Job drawing, mm, ordinate dimensions from the low corner. One solid piece. Round coordinates to 2 decimals unless told otherwise and drop trailing zeros. Order: outer loops, then holes, each group sorted by start corner. A loop starts at its lowest first (then second) coordinate and runs counter-clockwise, first axis right, second up. Notation, with made-up numbers: (62, 73.25) -> (96, 73.25) arc R7 cw to (96, 84.25) -> close; hole circle Ø10 at (52.5, 32.5). An arc over 180 degrees is marked (long way). Write item = value, one per line.
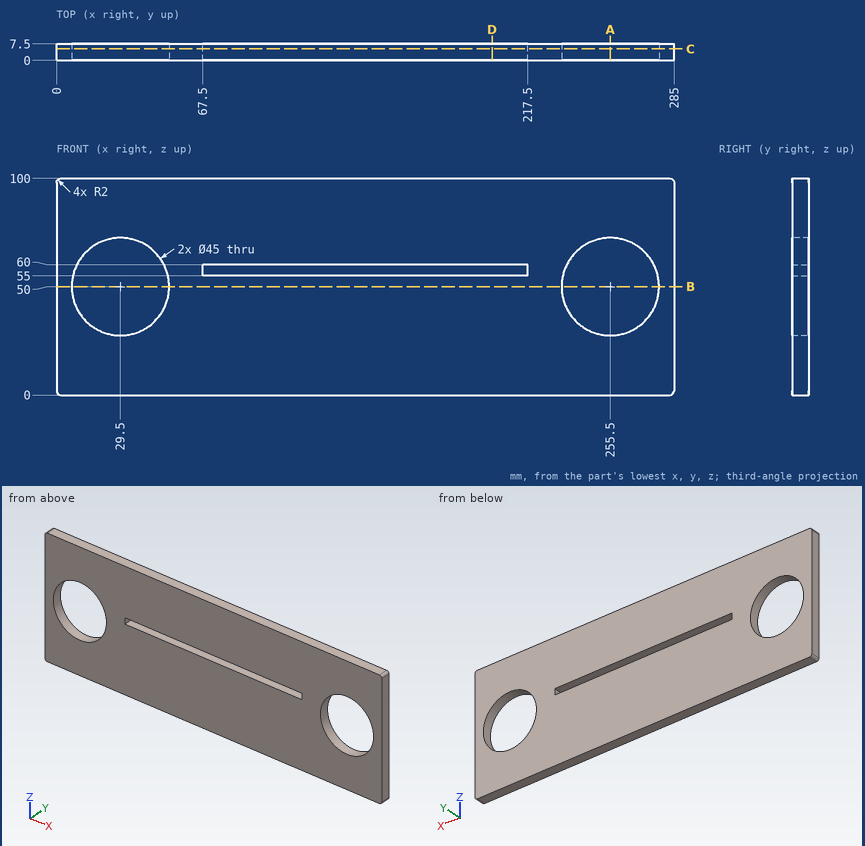
Q1. Cut at A-A, the plane x = 255.5. List the corners of the cut face in (y, z).
Check values:
outline = (0, 0) -> (7.5, 0) -> (7.5, 27.5) -> (0, 27.5) -> close; (0, 72.5) -> (7.5, 72.5) -> (7.5, 100) -> (0, 100) -> close
Q2. Cut at D-D, the plane x = 201. List the corners of the cut face in (y, z).
Check values:
outline = (0, 0) -> (7.5, 0) -> (7.5, 55) -> (0, 55) -> close; (0, 60) -> (7.5, 60) -> (7.5, 100) -> (0, 100) -> close
Q3. Probe probe 1 along X at (y, z) = (3.25, 50); probe 2 along Z at (x, y) = (256.5, 5.75); probe 3 along Z at (x, y) = (75.5, 3.5). List the from-to ranges inside material, lowest first.
Check values:
probe_1 = 0 to 7, 52 to 233, 278 to 285
probe_2 = 0 to 27.52, 72.48 to 100
probe_3 = 0 to 55, 60 to 100
Q4. Cut at C-C, the plane y = 5.25. List the corners of the cut face in (x, z).
Check values:
outline = (0, 2) arc R2 ccw to (2, 0) -> (283, 0) arc R2 ccw to (285, 2) -> (285, 98) arc R2 ccw to (283, 100) -> (2, 100) arc R2 ccw to (0, 98) -> close; hole circle Ø45 at (29.5, 50); hole (67.5, 55) -> (217.5, 55) -> (217.5, 60) -> (67.5, 60) -> close; hole circle Ø45 at (255.5, 50)
Q5. Cut at B-B, the plane z = 50. List the corners of the cut face in (x, y), and give its area (3 significant figures).
Check values:
outline = (0, 0) -> (7, 0) -> (7, 7.5) -> (0, 7.5) -> close; (52, 0) -> (233, 0) -> (233, 7.5) -> (52, 7.5) -> close; (278, 0) -> (285, 0) -> (285, 7.5) -> (278, 7.5) -> close
area = 1,460 mm²
